CAD build for the part. Positions are in the model's coordinates, mm. Face numbers are marked on the shaded views. A direction names the side the tool comes from. Give positions to 0.01 mm unless a question says otherwise; leave off trailing zeros. Loops run counter-clockwise (first coordinate to the right, second up) from the corner with the lowest first, then second, coordinate; pieces in that order, holes last. Notation, with made-up numbers: M -37.5,30 L 1.5,30 A15 cw 1.5,44 Z; hole C -24.75,76.25 d11. An arc over 180 degrees is marked long. Answer as CSV lines item,"result".
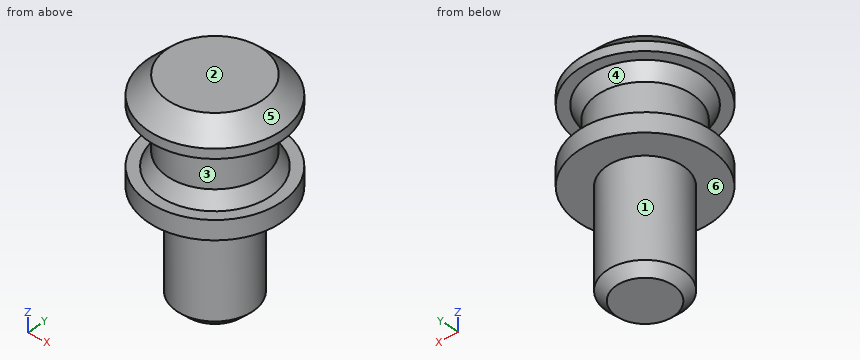
```python
from build123d import *

# Parameters (mm, degrees)
F2_SIZE = 2
F3_SIZE = 1


with BuildPart() as f1:
    # F0 (on Front) → F1 (revolve)
    with BuildSketch(Plane.XZ):
        Polygon((0, 11), (0, -11.235857), (4, -11.235857), (4, 0), (7, 0), (7, 2), (5.866025, 2), (5, 3.5), (5, 6.5), (5.866025, 8), (7, 8), (7, 11), align=None)
    revolve(axis=Axis((0, 0, -0.117929), (0, 0, -1)))

    # F2
    f2_edges = [f1.edges().sort_by_distance(p)[0] for p in [
        (-7, 0, 11),
    ]]
    chamfer(f2_edges, length=F2_SIZE)

    # F3
    f3_edges = [f1.edges().sort_by_distance(p)[0] for p in [
        (-4, 0, -11.235857),
    ]]
    chamfer(f3_edges, length=F3_SIZE)


solid = f1.part
```
Q1. Mould opens along Z. For the marked faces 4, 5 and 6 say: released by +Z, released by -Z, zero draft, split by the parting line, or undercut.
Solution:
face 4,"undercut"
face 5,"released by +Z"
face 6,"released by -Z"
Q2. Which spindle directions (+Z, -Z, +X, -X, +Y, -Y) get a long thin tool onto all of the face, cutting with end or side? Do the marked faces 1, 2 and 3. Say none if no direction does.
Solution:
face 1,"-Z"
face 2,"+Z, +X, -X, +Y, -Y"
face 3,"none"
Q3. Wall check: line 1 (Z direction, x = -5.25, y = -3.75); line 2 (Z direction, x = 4.5, y = -4); line 3 (Z direction, x = 3.25, y = -3). Give the ranges that are in metal, low to high. Write a range as [from, to].
Solution:
line 1,"z = [0, 2], [8, 9.55]"
line 2,"z = [0, 2], [8, 9.98]"
line 3,"z = [0, 11]"
Q4. Cut at D-D (z = -3). Write the cut outline in (x, y), and give its area (3 significant figures).
Solution:
outline,"C 0,0 d8"
area,"50.3 mm²"
Q5. Cut at A-A (x = 0). Write the cut outline in (y, z).
Solution:
outline,"M -7,0 L -4,0 L -4,-10.24 L -3,-11.24 L 3,-11.24 L 4,-10.24 L 4,0 L 7,0 L 7,2 L 5.87,2 L 5,3.5 L 5,6.5 L 5.87,8 L 7,8 L 7,9 L 5,11 L -5,11 L -7,9 L -7,8 L -5.87,8 L -5,6.5 L -5,3.5 L -5.87,2 L -7,2 Z"
Q6. Cut at C-C (z = 8.5). Write the cut outline in (x, y), and give its area (3 significant figures).
Solution:
outline,"C 0,0 d14"
area,"154 mm²"
Q7. Pin check, flat tips, straight feed: P1, Ø2, axis at x = -4.5, z = -3.5, coming from the +Y side; P2, Ø8, axis at y = -4.5, z = 4, coming from the +X side; P3, Ø1, axis at y = -1.5, z = 6, coming from the +X side. Stop position of each tip, or through.
Solution:
P1,"stops at y = 1.94"
P2,"stops at x = 6.92"
P3,"stops at x = 4.9"
